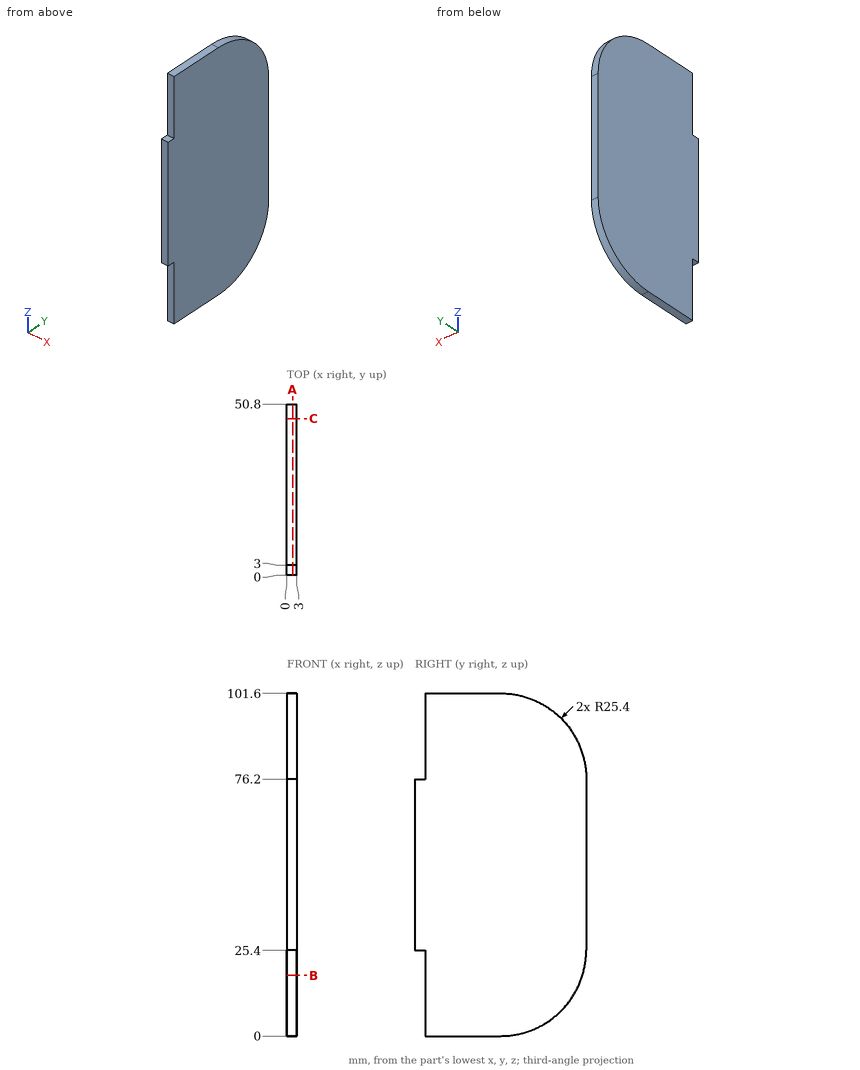
Geometry check sheet. Reference: drawing and pictorial views, mm from the part's lowest x, y, z. Round coordinates to 2 decimals unless told otherwise and drop trailing zeros. Loops run counter-clockwise (first coordinate to the right, second up) from the corner with the lowest first, then second, coordinate; pieces in that order, holes last. Notation, with made-up numbers: (25.5, 64.5) - (47.5, 64.5) arc R11 cw to (47.5, 69.5) - close; hole circle Ø11 at (27.25, 69). An arc over 180 degrees is marked (long way). One line per question, with ' | ' between items. Start each with the question number.
1. Cross-section at C-C on y = 46.5. Record the cut outline in (x, z), then the cut area to 3 significant figures.
2. Cross-section at B-B on z = 18. Record the cut outline in (x, y), then the cut area to 3 significant figures.
3. Depth check by flat-ended pin: pin 1 (1 mm diameter, centred on x = 1, y = 36.5, fed in from -Z); pin 2 (1.5 mm diameter, centred on x = 1.5, z = 19, fed in from -Y). Enter the tip coordinate at first touch or a pass-through.
4. Scan lines: line 1 (Z direction, x = 0.85, y = 48); line 2 (Y direction, x = 0.55, z = 82); line 3 (Z direction, x = 1.45, y = 43). Record each from-to range of solid material in increasing order. Write a range as [from, to].
5. Cross-section at A-A on x = 1.75. Record the cut outline in (y, z), then the cut area to 3 significant figures.
Taken from the geometry:
1) outline: (0, 11.26) - (3, 11.26) - (3, 90.34) - (0, 90.34) - close | area: 237 mm²
2) outline: (0, 3) - (3, 3) - (3, 49.7) - (0, 49.7) - close | area: 140 mm²
3) pin 1: z = 2.32 | pin 2: y = 3
4) line 1: [13.81, 87.79] | line 2: [3, 50.13] | line 3: [7.09, 94.51]
5) outline: (0, 25.4) - (3, 25.4) - (3, 0) - (25.4, 0) arc R25.4 ccw to (50.8, 25.4) - (50.8, 76.2) arc R25.4 ccw to (25.4, 101.6) - (3, 101.6) - (3, 76.2) - (0, 76.2) - close | area: 4,730 mm²
